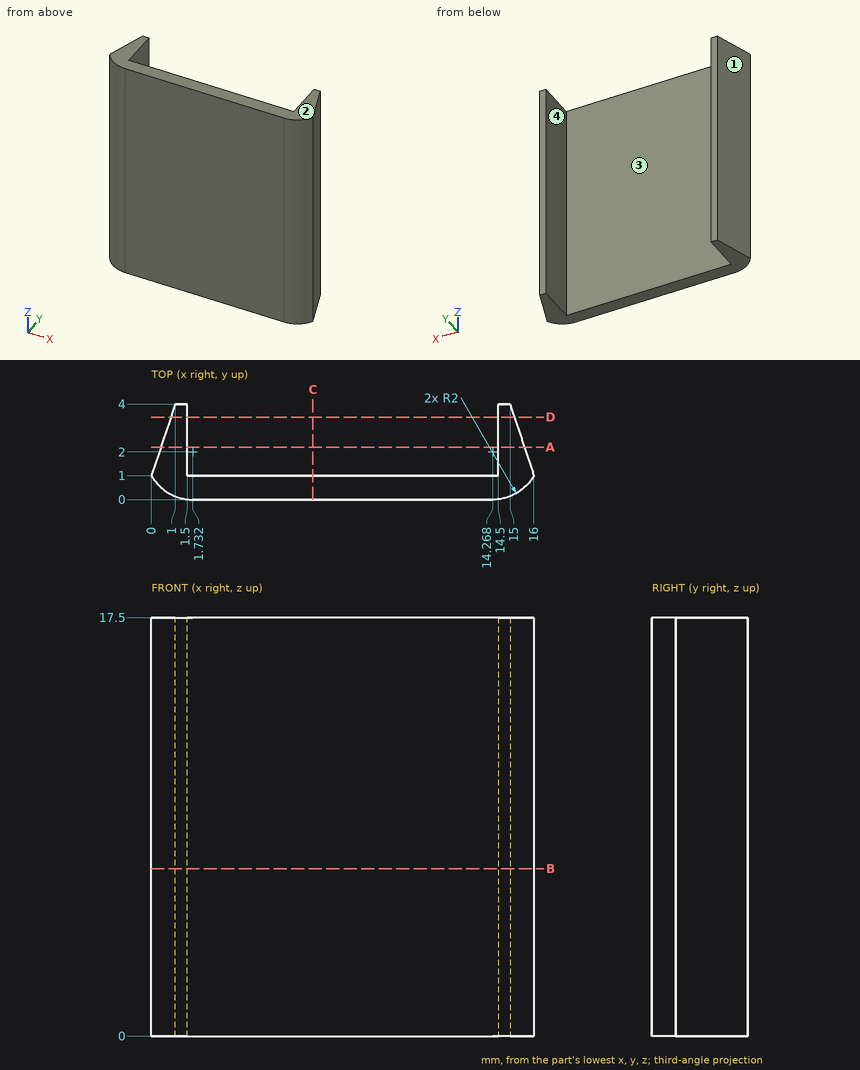
Source: three-view drawing plus pictorial views. Frame: mm from the lowest corner of the part. Round coordinates to 2 decimals unless told otherwise and drop trailing zeros. Loops run counter-clockwise (first coordinate to the right, second up) from the corner with the lowest first, then second, coordinate; pieces in that order, holes last.
Q1. Section C-C, the plane x = 6.75. Return loops of the section in (y, z), plus the area to 3 significant figures.
Q2. Section A-A, the plane y = 2.2. Return loops of the section in (x, z).
Q3. Mould query, pull axis X, two halves, no side actions, for the marked faces 1, 2, 3 and 4. Classes: pulls with the +X half, pulls with the -X half, needs draft (parallel to the pull), parting line crosses it, or undercut.
Q4. Ray query, line 1 (Y direction, x = 12.5, z = 4.5); line 2 (X direction, y = 3.6, z = 14.75); line 3 (X direction, y = 2.7, z = 15.5). Return the intervals inside material, ascending.
Q5. Section B-B, the plane z = 7. Return loops of the section in (x, y), plus the area to 3 significant figures.
Q6. Section D-D, the plane y = 3.45. Return loops of the section in (x, z).
Q7. First-contact query: P1, Ø1.5, axis at y = 3, z = 7, coming from the -X side; P2, Ø1.5, axis at y = 2, z = 12.5, coming from the -X side; P3, Ø6.5, axis at x = 9, z = 8.5, coming from the +Y side. Flat tips, straight axial feed; report the tip coordinate or a pass-through.
Solutions:
1. outline: (0, 0) - (1, 0) - (1, 17.5) - (0, 17.5) - close
1. area: 17.5 mm2
2. outline: (0.4, 0) - (1.5, 0) - (1.5, 17.5) - (0.4, 17.5) - close; (14.5, 0) - (15.6, 0) - (15.6, 17.5) - (14.5, 17.5) - close
3. face 1: pulls with the -X half
3. face 2: needs draft
3. face 3: undercut
3. face 4: undercut
4. line 1: y = 0 to 1
4. line 2: x = 0.87 to 1.5, 14.5 to 15.13
4. line 3: x = 0.57 to 1.5, 14.5 to 15.43
5. outline: (0, 1) arc R2 ccw to (1.73, 0) - (14.27, 0) arc R2 ccw to (16, 1) - (15, 4) - (14.5, 4) - (14.5, 1) - (1.5, 1) - (1.5, 4) - (1, 4) - close
5. area: 21.0 mm2
6. outline: (0.82, 0) - (1.5, 0) - (1.5, 17.5) - (0.82, 17.5) - close; (14.5, 0) - (15.18, 0) - (15.18, 17.5) - (14.5, 17.5) - close
7. P1: stops at x = 0.42
7. P2: stops at x = 0.08
7. P3: stops at y = 1
